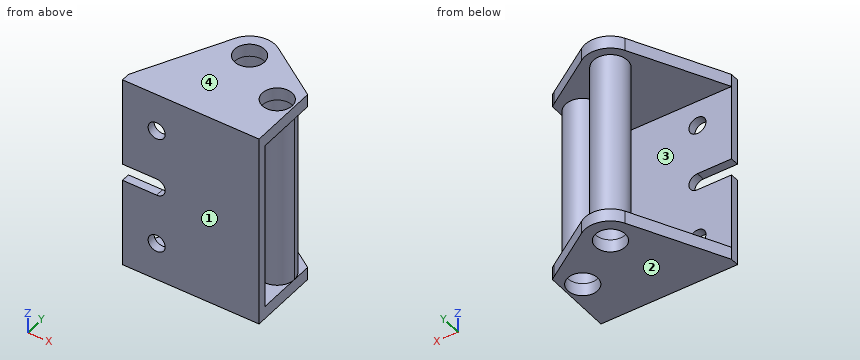
Autodesk Inventor part; units mm, degrees
ref_plane "YZ Plane" through (0, 0, 0) normal (1, 0, 0) x (0, 1, 0)
ref_plane "XZ Plane" through (0, 0, 0) normal (0, 1, 0) x (-1, 0, 0)
ref_plane "XY Plane" through (0, 0, 0) normal (0, 0, 1) x (1, 0, 0)
sketch "Sketch1" plane through (0, 0, 0) normal (0, 1, 0) x (-1, 0, 0)
  line L0 (0, 0) -> (-76.2, 0)
  line L1 (-76.2, 0) -> (-76.2, -63.5) construction
  line L2 (-76.2, -63.5) -> (0, -63.5)
  line L3 (0, -63.5) -> (0, 0) construction
  line L4 (0, -31.75) -> (44.45, -31.75) construction
  line L5 (-76.2, -31.75) -> (-127, -31.75) construction
  circle A0 centre (44.45, -31.75) radius 3.175
  circle A1 centre (-127, -31.75) radius 3.175 construction
  circle A2 centre (-114.3, -31.75) radius 3.175 construction
  line L6 (-114.3, -34.925) -> (-127, -34.925)
  line L7 (-114.3, -28.575) -> (-127, -28.575)
  arc A3 (-114.3, -34.925) -> (-114.3, -28.575) centre (-114.3, -31.75) ccw
  arc A4 (-127, -28.575) -> (-127, -34.925) centre (-127, -31.75) ccw
  line L8 (0, -63.5) -> (47.5152, -37.3112)
  line L9 (47.5152, -26.1888) -> (0, 0)
  line L10 (-76.2, -63.5) -> (-129.7757, -37.4612)
  line L11 (-129.7757, -26.0388) -> (-76.2, 0)
  arc A5 (47.5152, -37.3112) -> (47.5152, -26.1888) centre (44.45, -31.75) ccw
  arc A6 (-129.7757, -26.0388) -> (-129.7757, -37.4612) centre (-127, -31.75) ccw
  circle A7 centre (-76.2, -31.75) radius 3.175 construction
  circle A8 centre (-63.5, -31.75) radius 3.175 construction
  line L12 (-76.2, -28.575) -> (-63.5, -28.575) construction
  line L13 (-76.2, -34.925) -> (-63.5, -34.925) construction
  line L14 (-63.5, -28.575) -> (-76.2, -28.575)
  line L15 (-76.2, -34.925) -> (-63.5, -34.925)
  arc A9 (-63.5, -34.925) -> (-63.5, -28.575) centre (-63.5, -31.75) ccw
  arc A10 (-76.2, -28.575) -> (-76.2, -34.925) centre (-76.2, -31.75) ccw
  circle A11 centre (0, -31.75) radius 3.175 construction
  circle A12 centre (-12.7, -31.75) radius 3.175 construction
  line L16 (0, -28.575) -> (-12.7, -28.575) construction
  line L17 (0, -34.925) -> (-12.7, -34.925) construction
  arc A13 (-12.7, -28.575) -> (-12.7, -34.925) centre (-12.7, -31.75) ccw
  arc A14 (0, -34.925) -> (0, -28.575) centre (0, -31.75) ccw
  line L18 (-12.7, -34.925) -> (0, -34.925)
  line L19 (-12.7, -28.575) -> (0, -28.575)
  dimension "d0" = 76.2
  dimension "d1" = 63.5
  dimension "d2" = 44.45
  dimension "d3" = 50.8
  dimension "d4" = 6.35
  dimension "d5" = 6.35
  dimension "d6" = 6.35
  dimension "d7" = 12.7
  dimension "d8" = 6.35
  dimension "d9" = 0
  dimension "d10" = 0
  dimension "d11" = 0
  dimension "d12" = 0
  dimension "d13" = 6.35
  dimension "d14" = 6.35
  dimension "d15" = 12.7
  dimension "d16" = 0
  dimension "d17" = 6.35
  dimension "d18" = 6.35
  dimension "d19" = 0
  dimension "d20" = 12.7
extrude "Extrusion1" add sketch "Sketch1" along normal blind 3.175
sketch "Sketch2" plane through (0, 0, 0) normal (0, 0, 1) x (1, 0, 0)
  line L0 (0, 0) -> (76.2, 0)
  line L1 (76.2, 0) -> (76.2, 3.175)
  line L2 (0, 3.175) -> (76.2, 3.175)
  line L3 (0, 0) -> (0, 3.175)
  circle A0 centre (25.4, 31.75) radius 5.5562
  circle A1 centre (44.45, 19.05) radius 5.5563
  line L4 (0, 3.175) -> (16.9289, 36.1049)
  line L5 (30.6835, 39.6753) -> (49.7335, 26.9753)
  line L6 (50.8395, 26.114) -> (76.2, 3.175)
  arc A2 (30.6835, 39.6753) -> (16.9289, 36.1049) centre (25.4, 31.75) ccw
  arc A3 (50.8395, 26.114) -> (49.7335, 26.9753) centre (44.45, 19.05) ccw
  dimension "d23" = 11.1125
  dimension "d24" = 31.75
  dimension "d25" = 25.4
  dimension "d26" = 11.1125
  dimension "d27" = 19.05
  dimension "d28" = 31.75
  dimension "d29" = 9.525
extrude "Extrusion2" add sketch "Sketch2" along normal blind 4.7625
sketch "Sketch3" plane through (76.2, 0, -63.5) normal (0, 0, -1) x (-1, 0, 0)
  line L0 (0, 0) -> (76.2, 0)
  line L1 (76.2, 0) -> (76.2, 3.175)
  line L2 (0, 3.175) -> (76.2, 3.175)
  line L3 (0, 0) -> (0, 3.175)
  line L4 (59.2711, 36.1049) -> (76.2, 3.175)
  arc A0 (59.2711, 36.1049) -> (45.5165, 39.6753) centre (50.8, 31.75) ccw
  line L5 (26.4665, 26.9753) -> (45.5165, 39.6753)
  arc A1 (26.4665, 26.9753) -> (25.3605, 26.114) centre (31.75, 19.05) ccw
  line L6 (0, 3.175) -> (25.3605, 26.114)
  circle A2 centre (31.75, 19.05) radius 5.5563
  circle A3 centre (50.8, 31.75) radius 5.5562
  line L7 (76.2, 0) -> (0, 0)
  line L8 (0, 0) -> (0, 3.175)
  line L9 (76.2, 3.175) -> (76.2, 0)
extrude "Extrusion3" add sketch "Sketch3" along normal blind 4.7625
sketch "Sketch5" plane through (0, 0, 0) normal (0, 0, -1) x (-1, 0, 0)
  line L0 (0, 3.175) -> (-76.2, 3.175)
  line L1 (-16.9289, 36.1049) -> (0, 3.175)
  arc A0 (-16.9289, 36.1049) -> (-30.6835, 39.6753) centre (-25.4, 31.75) ccw
  line L2 (-49.7335, 26.9753) -> (-30.6835, 39.6753)
  arc A1 (-49.7335, 26.9753) -> (-50.8395, 26.114) centre (-44.45, 19.05) ccw
  line L3 (-76.2, 3.175) -> (-50.8395, 26.114)
  circle A2 centre (-44.45, 19.05) radius 5.5563
  circle A3 centre (-25.4, 31.75) radius 5.5562
  circle A4 centre (-44.45, 19.05) radius 6.35
  circle A5 centre (-25.4, 31.75) radius 6.35
  point P0 (0, 0)
  dimension "d38" = 12.7
  dimension "d39" = 12.7
extrude "Extrusion5" add sketch "Sketch5" along normal blind 63.5 contours A4 | A5
sketch "Sketch6" plane through (0, 3.175, 0) normal (0, 1, 0) x (1, 0, 0)
  line L0 (0, 34.925) -> (12.7, 34.925)
  arc A0 (12.7, 28.575) -> (12.7, 34.925) centre (12.7, 31.75) ccw
  line L1 (12.7, 28.575) -> (0, 28.575)
  arc A1 (0, 34.925) -> (0, 28.575) centre (0, 31.75) ccw
  arc A2 (63.5, 34.925) -> (63.5, 28.575) centre (63.5, 31.75) ccw
  line L2 (63.5, 34.925) -> (76.2, 34.925)
  arc A3 (76.2, 28.575) -> (76.2, 34.925) centre (76.2, 31.75) ccw
  line L3 (76.2, 28.575) -> (63.5, 28.575)
  arc A4 (127, 28.575) -> (127, 34.925) centre (127, 31.75) ccw
  line L4 (127, 28.575) -> (114.3, 28.575)
  arc A5 (114.3, 34.925) -> (114.3, 28.575) centre (114.3, 31.75) ccw
  line L5 (114.3, 34.925) -> (127, 34.925)
  circle A6 centre (-44.45, 31.75) radius 3.175
  line L6 (0, 0) -> (76.2, 0)
  line L7 (76.2, 0) -> (129.7757, 26.0388)
  arc A7 (129.7757, 26.0388) -> (129.7757, 37.4612) centre (127, 31.75) ccw
  line L8 (129.7757, 37.4612) -> (76.2, 63.5)
  line L9 (76.2, 63.5) -> (0, 63.5)
  line L10 (0, 63.5) -> (-47.5152, 37.3112)
  arc A8 (-47.5152, 37.3112) -> (-47.5152, 26.1888) centre (-44.45, 31.75) ccw
  line L11 (-47.5152, 26.1888) -> (0, 0)
  circle A9 centre (88.9, 31.75) radius 3.175
  circle A10 centre (63.5, 9.525) radius 3.175
  circle A11 centre (63.5, 53.975) radius 3.175
  circle A12 centre (-12.7, 31.75) radius 3.175
  circle A13 centre (12.7, 9.525) radius 3.175
  circle A14 centre (12.7, 53.975) radius 3.175
  dimension "d42" = 6.35
  dimension "d43" = 6.35
  dimension "d44" = 6.35
  dimension "d45" = 6.35
  dimension "d46" = 6.35
  dimension "d47" = 6.35
  dimension "d50" = 22.225
  dimension "d51" = 22.225
  dimension "d52" = 0
  dimension "d53" = 0
  dimension "d54" = 0
  dimension "d55" = 12.7
  dimension "d56" = 12.7
  dimension "d57" = 0
  dimension "d58" = 0
  dimension "d59" = 0
  dimension "d60" = 22.225
  dimension "d61" = 22.225
extrude "Extrusion6" cut sketch "Sketch6" against normal blind 63.5 contours A9 | A10 | A11 | A12 | A13 | A14
sketch "Sketch7" plane through (0, 0, 0) normal (0, -1, 0) x (1, 0, 0)
  circle A0 centre (12.7, -9.525) radius 3.175
  circle A1 centre (63.5, -53.975) radius 3.175
  circle A2 centre (88.9, -31.75) radius 3.175
  circle A3 centre (63.5, -9.525) radius 3.175
  circle A4 centre (-12.7, -31.75) radius 3.175
  circle A5 centre (12.7, -53.975) radius 3.175
  line L0 (12.7, -34.925) -> (0, -34.925)
  arc A6 (0, -28.575) -> (0, -34.925) centre (0, -31.75) ccw
  line L1 (0, -28.575) -> (12.7, -28.575)
  arc A7 (12.7, -34.925) -> (12.7, -28.575) centre (12.7, -31.75) ccw
  arc A8 (63.5, -28.575) -> (63.5, -34.925) centre (63.5, -31.75) ccw
  line L2 (63.5, -28.575) -> (76.2, -28.575)
  arc A9 (76.2, -34.925) -> (76.2, -28.575) centre (76.2, -31.75) ccw
  line L3 (76.2, -34.925) -> (63.5, -34.925)
  arc A10 (127, -34.925) -> (127, -28.575) centre (127, -31.75) ccw
  line L4 (127, -34.925) -> (114.3, -34.925)
  arc A11 (114.3, -28.575) -> (114.3, -34.925) centre (114.3, -31.75) ccw
  line L5 (114.3, -28.575) -> (127, -28.575)
  circle A12 centre (-44.45, -31.75) radius 3.175
  line L6 (-47.5152, -26.1888) -> (0, 0)
  arc A13 (-47.5152, -26.1888) -> (-47.5152, -37.3112) centre (-44.45, -31.75) ccw
  line L7 (0, -63.5) -> (-47.5152, -37.3112)
  line L8 (129.7757, -37.4612) -> (76.2, -63.5)
  arc A14 (129.7757, -37.4612) -> (129.7757, -26.0388) centre (127, -31.75) ccw
  line L9 (76.2, 0) -> (129.7757, -26.0388)
  line L10 (76.2, 0) -> (76.2, 4.7625)
  line L11 (0, 4.7625) -> (76.2, 4.7625)
  line L12 (0, 0) -> (0, 4.7625)
  line L13 (76.2, 4.7625) -> (50.8, 4.7625) construction
  line L14 (0, 4.7625) -> (76.2, 4.7625) construction
  line L15 (50.8, 4.7625) -> (133.35, 4.7625)
  line L16 (133.35, 4.7625) -> (133.35, -71.4375)
  line L17 (133.35, -71.4375) -> (50.8, -71.4375)
  line L18 (50.8, -71.4375) -> (50.8, 4.7625)
  line L19 (0, -63.5) -> (0, -68.2625)
  line L20 (76.2, -68.2625) -> (0, -68.2625)
  line L21 (76.2, -63.5) -> (76.2, -68.2625)
  dimension "d64" = 25.4
  dimension "d65" = 82.55
  dimension "d66" = 76.2
extrude "Extrusion7" cut sketch "Sketch7" against normal blind 63.5 contours L11 L10 L9 A14 L8 L21 L20 L18 | L15 L16 A14 L9 L10 | L20 L21 L8 A14 L16 L17 L18
sketch "Sketch8" plane through (0, 3.175, 0) normal (0, 1, 0) x (1, 0, 0)
  circle A0 centre (-44.45, 31.75) radius 3.175
  circle A1 centre (-12.7, 31.75) radius 3.175
  line L0 (0, 63.5) -> (-63.5, 63.5)
  line L1 (-63.5, 63.5) -> (-63.5, 0)
  line L2 (-63.5, 0) -> (0, 0)
  line L3 (0, 0) -> (0, 63.5)
  dimension "d69" = 63.5
  dimension "d70" = 63.5
extrude "Extrusion8" cut sketch "Sketch8" against normal blind 25.4
properties part number "garage door hinge" material "Aluminum 6061"
Verification items for the finished model (mm, model axes). Face numbers are marked on the shaded views. Give positions to 0.01 mm unless a question says otherwise; leave off trailing zeros. Write each loop counter-clockwise with the first axis right and the second up, starting at its lowest first coordinate (ties: lowest second). Pieces come first, ordered by that corner, then holes. Notation, with made-up numbers: M 71.5,-25.75 L 111.5,-25.75 A16 cw 111.5,-7.75 Z; hole C 51,38 d10. An arc over 180 degrees is marked long. Write item = value, one per line.
(1) Material ranges on line 1 (Y direction, x = 25, z = -19) (3 decimals); line 2 (Z direction, x = 34.5, y = 21.5); line 3 (Y direction, x = 42, z = -33) (3 decimals), recorded low to high.
Found:
line_1 = 0 to 3.175, 25.413 to 26.208, 37.292 to 38.087
line_2 = -68.26 to -63.5, 0 to 4.76
line_3 = 0 to 3.175, 13.192 to 14.063, 24.037 to 24.908
(2) Sectioned sample at C-C (y = 23). Record the cut outline in (x, z), then the cut area to 3 significant figures.
Found:
outline = M 10.19,-68.26 L 40.54,-68.26 L 40.54,4.76 L 10.19,4.76 L 10.19,0 L 39.48,0 L 39.48,-63.5 L 10.19,-63.5 Z; M 48.36,-68.26 L 50.8,-68.26 L 50.8,-63.5 L 49.42,-63.5 L 49.42,0 L 50.8,0 L 50.8,4.76 L 48.36,4.76 Z
area = 448 mm2
(3) Go/stop test with flat-tipped pins: pin 1 Ø5 at (x, z) = (35, -26) entering from -Y; pin 2 Ø8.5 at (x, z) = (12.7, -53.975) entering from +Y (3 decimals); pin 3 Ø5 at (y, z) = (36, -32.5) entering from +X; pin 4 Ø1 at (y, z) = (24, -57) entering from -X. Record where each tip stops, or that it passes through.
Found:
pin_1 = 0
pin_2 = 3.175
pin_3 = 31.5
pin_4 = 39.92
(4) Draft check along Z on the marked faces 1, 2, 3 and 4. Enter one of: released by +Z, released by -Z, zero draft, split by the parting line, or undercut.
Found:
face_1 = zero draft
face_2 = released by -Z
face_3 = undercut
face_4 = released by +Z
(5) Sectioned sample at D-D (z = -40). Record the cut outline in (x, y) (3 decimals).
Found:
outline = M 0,0 L 50.8,0 L 50.8,3.175 L 0,3.175 Z; C 25.4,31.75 d12.7; C 44.45,19.05 d12.7; hole C 25.4,31.75 d11.112; hole C 44.45,19.05 d11.113
(6) Sectioned sample at B-B (z = -31.75). Record the cut outline in (x, y) (3 decimals).
Found:
outline = M 15.875,0 L 50.8,0 L 50.8,3.175 L 15.875,3.175 Z; C 25.4,31.75 d12.7; C 44.45,19.05 d12.7; hole C 25.4,31.75 d11.112; hole C 44.45,19.05 d11.113
(7) Sectioned sample at A-A (x = 25.4). Record the cut outline in (y, z) (1 decimal).
Found:
outline = M 0,-68.3 L 26.2,-68.3 L 26.2,4.8 L 0,4.8 Z; M 37.3,-68.3 L 41.3,-68.3 L 41.3,-63.5 L 38.1,-63.5 L 38.1,0 L 41.3,0 L 41.3,4.8 L 37.3,4.8 Z; hole M 3.2,-63.5 L 25.4,-63.5 L 25.4,0 L 3.2,0 Z
